Here's how the part is built. I have some questions about the finished solid (model axes, mm). A direction names the side the tool comes from. Round coordinates to 2 decimals unless told otherwise and drop trailing zeros. Order: outer loops, then holes, each group sorted by start corner. A loop starts at its lowest first (then second) coordinate and runs counter-clockwise, first axis right, second up. Notation, with made-up numbers: M 79.5,-27.5 L 83.5,-27.5 A21 cw 83.5,-22.5 Z; hole C 14,46 d7. An arc over 180 degrees is marked long. Use one line per item in the form item = value. Start each with the question number.
```python
from build123d import *

# Parameters (mm, degrees)
BOSS_EXTRUDE1_DEPTH         = 2
SKETCH3_W                   = 4.004504799
SKETCH3_H                   = 7.007808652
SKETCH3_W_2                 = 4
SKETCH3_H_2                 = 5
CUT_EXTRUDE1_DEPTH          = 10
SKETCH4_R                   = 20
CUT_EXTRUDE2_DEPTH          = 1
F_3_0MM_PRESS_DOWEL_HOLE1_D = 3
CUT_EXTRUDE3_DEPTH          = 272.480461976


with BuildPart() as part:
    # Sketch1 → Boss-Extrude1 (new body)
    with BuildSketch(Plane.XY):
        Polygon((-70, 100), (-70, -72.799540117), (70, -72.799540117), (70, 44.524791386), (-26.08587988, 100), align=None)
    extrude(amount=BOSS_EXTRUDE1_DEPTH)

    # Sketch3 → Cut-Extrude1 (cut)
    with BuildSketch(Plane.XY.offset(2)):
        with Locations((21.429491924, 36.193920339)):
            Rectangle(SKETCH3_W, SKETCH3_H)
        with Locations((-64, 78.155444566)):
            Rectangle(SKETCH3_W_2, SKETCH3_H_2)
        Polygon((-14.572335871, -75.184527756), (23.015368961, -75.184527756), (23.015368961, -31.503722023), (19.595167527, -22.106795815), (-17.992537304, -35.787601548), (-14.572335871, -45.184527756), align=None)
    extrude(amount=-CUT_EXTRUDE1_DEPTH, mode=Mode.SUBTRACT)

    # Sketch4 → Cut-Extrude2 (cut)
    with BuildSketch(Plane.XY.offset(2)):
        with Locations((-41.723720558, 72.655444566)):
            Circle(SKETCH4_R)
    extrude(amount=-CUT_EXTRUDE2_DEPTH, mode=Mode.SUBTRACT)

    # Ø3.0mm Press Dowel Hole1 (through all)
    with Locations(Plane(origin=(-89.742029537, -119.499715795, 0), x_dir=(-1, 0, 0), z_dir=(0, 0, -1))):
        with Locations((-23.542258378, 99.781049413), (-25.594379238, 52.014538143), (-70.699625036, 68.431505023), (-70.526889417, 116.882056579), (-111.491838386, 131.259989766), (-119.586439667, 85.314281565), (-155.294759257, 98.311047011), (-152.806439447, 156.481766603), (-65.878236217, 157.017664987), (-102.576966028, 185.481766603), (-52.347492608, 214.481766603), (-25.242029537, 178.499715795)):
            Hole(F_3_0MM_PRESS_DOWEL_HOLE1_D / 2)

    # Sketch7 → Cut-Extrude3 (cut, through all)
    with BuildSketch(Plane(origin=(-89.742029537, -119.499715795, 2), x_dir=(1, 0, 0), z_dir=(0, 0, 1))):
        with BuildLine():
            Line((44.742029537, 154.499715795), (44.742029537, 124.499715795))
            ThreePointArc((44.742029537, 124.499715795), (39.742029537, 119.499715795), (34.742029537, 124.499715795))
            Line((34.742029537, 124.499715795), (34.742029537, 154.499715795))
            ThreePointArc((34.742029537, 154.499715795), (39.742029537, 159.499715795), (44.742029537, 154.499715795))
        make_face()
    extrude(amount=-CUT_EXTRUDE3_DEPTH, mode=Mode.SUBTRACT)


solid = part.part
```
1) If we section it at C-C on x = 49: Write out the boundary of the cut face in (y, z).
2) If we section it at D-D on x = 8: Write out the boundary of the cut face in (y, z).
3) If we section it at A-A on y = -56: Write out the boundary of the cut face in (x, z), then the cut area to 3 significant figures.
4) If I drill on line 1 (X direction, y = -51, z = 0.3); line 2 (Y direction, x = -64.5, z = 1.15); line 3 (X direction, y = 79, z = 0.2), over which ranges is the centre line in solid material (lowest first)?
5) Will these pins go through, and if not, where does the flat tip stop? pin 1 Ø12 at (x, y) = (-35.5, 70) entering from +Z; pin 2 Ø0.6 at (x, z) = (21, 0.5) entering from +Y; pin 3 Ø1 at (x, z) = (-4, 1) entering from +Y.
6) If we section it at B-B on z = 1.5: Give the number of separate pieces and of enclosed holes in the cut face, then the cut area to 3 significant figures.
7) On a 3-axis mill with a long thin cutter (end or side, diameter ignored), from which of +Z, -Z, +X, -X, +Y, -Y can I reach the whole of each face in a straight line? I mean faces 4 (the flat face through (-1, 15, 0)), 5 (the flat face through (21.33, -26.87, 1.01)), 6 (the cylindrical face through (-50, 40, 1)), 7 (the cylindrical face through (-22.647, 78.663, 1.507)). Say none if no direction works.
8) If we mould it in two halves opening along X, with no side actions, what happens to faces 1 (the cylindrical face through (-50, 0, 1)), 2 (the flat face through (-1, 15, 2)), 3 (the flat face through (22.63, 71.874, 0.986))? For each: +X half, -X half, draft (parallel to the pull), parting line (faces both ways), or undercut.
Completed:
q1.outline = M -72.8,0 L 56.65,0 L 56.65,2 L -72.8,2 Z
q2.outline = M -26.33,0 L 80.32,0 L 80.32,2 L -26.33,2 Z
q3.outline = M -70,0 L -14.57,0 L -14.57,2 L -70,2 Z; M 23.02,0 L 70,0 L 70,2 L 23.02,2 Z
q3.area = 205 mm²
q4.line_1 = -70 to -20.54, -17.54 to -14.57, 23.02 to 70
q4.line_2 = -72.8 to -68.94, -66.03 to 57.5, 60.5 to 75.66, 80.66 to 100
q4.line_3 = -70 to -66, -62 to 10.29
q5.pin_1 = 1
q5.pin_2 = 72.99
q5.pin_3 = 87.54
q6.separate_pieces = 1
q6.enclosed_holes = 16
q6.area = 18,100 mm²
q7.face_4 = -Z, +X, -X, +Y, -Y
q7.face_5 = +Z, -Z, -Y
q7.face_6 = +Z, -Z
q7.face_7 = +Z
q8.face_1 = undercut
q8.face_2 = draft
q8.face_3 = +X half
